from build123d import *

# Parameters (mm, degrees)
F0_R          = 1.55
F1_DEPTH      = 3
F2_SIZE2      = 2.99999
F2_SIZE       = 0.49999
F2_2_SIZE2    = 2.99999
F2_2_SIZE     = 0.49999
F4_DEPTH      = 6
F5_DEPTH      = 6
F6_R          = 1.5
F7_DEPTH      = 25
F9_W          = 5.3
F9_H          = 30.2732266598
F10_DEPTH     = 25
F11_R         = 4
F12_T4_DEPTH  = 20.5670004785
F12_T10_DEPTH = 20.5670004785
F12_T16_DEPTH = 20.5670004785
F12_T22_DEPTH = 20.5670004785
F13_SIZE      = 0.2


# Not quite as in the source:
# - a fillet or chamfer that OpenCascade refuses, or shapes differently, is made with other operations: its cross-section is extruded or revolved along the edge and cut away or added
# - a fillet or chamfer is up to 0.001 mm smaller than in the source, because OpenCascade refuses the exact size
# - ends of sketch curves that miss each other by under 0.0002 mm in the source are joined


with BuildPart() as f1:
    # F0 (on Front) → F1 (new body)
    with BuildSketch(Plane.XZ):
        with BuildLine():
            Line((-17.1, 5.6), (-17.1, -5.6))
            Line((-17.1, -5.6), (17.1, -5.6))
            Line((17.1, -5.6), (17.1, 5.6))
            Line((17.1, 5.6), (9.1844569534, 5.6))
            add(Edge.make_bspline(
                [(9.1844569534, 5.6), (9.1844569534, 2.9670004785), (9.1844569534, 2.9670004785), (-0.0155430466, 2.9670004785)],
                knots=[0, 0, 0, 0, 9.5693619495, 9.5693619495, 9.5693619495, 9.5693619495], degree=3))
            add(Edge.make_bspline(
                [(-9.2155430466, 5.6), (-9.2155430466, 2.9670004785), (-9.2155430466, 2.9670004785), (-0.0155430466, 2.9670004785)],
                knots=[0, 0, 0, 0, 9.5693618638, 9.5693618638, 9.5693618638, 9.5693618638], degree=3))
            Line((-9.2155430466, 5.6), (-17.1, 5.6))
        make_face()
        with Locations((-13, 0)):
            Circle(F0_R, mode=Mode.SUBTRACT)
        with Locations((13, 0)):
            Circle(F0_R, mode=Mode.SUBTRACT)
    extrude(amount=F1_DEPTH)

    # F2 (size 0.5 and 3 in the source; OpenCascade refuses exactly that, so slightly less here)
    f2_edges = [f1.edges().sort_by_distance(p)[0] for p in [
        (-13.157772, 0, 5.6),
        (13.142228, 0, 5.6),
    ]]
    f2_side = f1.faces().sort_by_distance((0.002222, 0, -0.619959))[0]
    chamfer(f2_edges, length=F2_SIZE, length2=F2_SIZE2, reference=f2_side)

    # F2#2 (size 0.5 and 3 in the source; OpenCascade refuses exactly that, so slightly less here)
    f2_2_edges = [f1.edges().sort_by_distance(p)[0] for p in [
        (0, -3, -5.6),
    ]]
    f2_2_side = f1.faces().sort_by_distance((0.002222, -3, -0.619959))[0]
    chamfer(f2_2_edges, length=F2_2_SIZE, length2=F2_2_SIZE2, reference=f2_2_side)

    # F3 (on Right) → F4 (join)
    with BuildSketch(Plane.YZ):
        Polygon((-33.2732266598, 2.4479631427), (-3, -5.1), (-3, 2.9670004785), (-4.2113326633, 3.2690196322), (-4.1453789697, 3.5335454488), (-31.3136593055, 10.3073585255), align=None)
    extrude(amount=F4_DEPTH)

    # F5 (add): a face of the model
    f5_faces = [f1.faces().sort_by_distance(p)[0] for p in [
        (0, -17.6712487641, 2.6798726591),
    ]]
    extrude(f5_faces, amount=F5_DEPTH)

    # F6 (on face) → F7 (cut)
    with BuildSketch(Plane.YZ.offset(6)):
        with Locations((-27.4419643513, 5.1680513561)):
            Circle(F6_R)
        with Locations((-17.7390070885, 2.7488324001)):
            Circle(F6_R)
        with Locations((-12.8875284571, 1.5392229221)):
            Circle(F6_R)
        with Locations((-8.0360498257, 0.3296134441)):
            Circle(F6_R)
    extrude(amount=-F7_DEPTH, mode=Mode.SUBTRACT)

    # F9 (on face) → F10 (cut)
    with BuildSketch(Plane(origin=(0, 0, -5.6), x_dir=(1, 0, 0), z_dir=(0, 0, -1))):
        with Locations((0, 18.1366133299)):
            Rectangle(F9_W, F9_H)
    extrude(amount=-F10_DEPTH, mode=Mode.SUBTRACT)

    # F11
    f11_edges = [f1.edges().sort_by_distance(p)[0] for p in [
        (-4.325, -33.273227, 2.447963),
        (4.325, -33.273227, 2.447963),
        (-4.325, -31.313659, 10.307359),
        (4.325, -31.313659, 10.307359),
    ]]
    fillet(f11_edges, radius=F11_R)

    # F12: fillet of radius 2.5 on 2 edges, made by hand


with BuildPart() as f12_tool2:
    # F12_s3 → F12_t4 (new body)
    with BuildSketch(Plane.XY.offset(-11.35)):
        with BuildLine():
            ThreePointArc((-0.15, -3), (-1.917766953, -3.732233047), (-2.65, -5.5))
            Line((-2.65, -5.5), (-2.65, -3))
            Line((-2.65, -3), (-0.15, -3))
        make_face()
    extrude(amount=F12_T4_DEPTH)

    split(bisect_by=Plane(origin=(0, 0.520882565, 2.0891458603), x_dir=(1, 0, 0), z_dir=(0, -0.2419218956, -0.9702957263)), keep=Keep.TOP)

    split(bisect_by=Plane(origin=(0, -1.3727310958, -5.505723706), x_dir=(1, 0, 0), z_dir=(0, 0.2419218956, 0.9702957263)), keep=Keep.TOP)


with BuildPart() as f1_1:
    add(f1.part)

    # F12_t1: union F12_tool2
    add(f12_tool2.part)


with BuildPart() as f12_tool8:
    # F12_s9 → F12_t10 (new body)
    with BuildSketch(Plane.XY.offset(-11.35)):
        with BuildLine():
            ThreePointArc((-0.15, -3), (-1.917766953, -3.732233047), (-2.65, -5.5))
            Line((-2.65, -5.5), (-2.65, -3))
            Line((-2.65, -3), (-0.15, -3))
        make_face()
    extrude(amount=F12_T10_DEPTH)

    split(bisect_by=Plane(origin=(0, -4.7322152283, 1.1798737719), x_dir=(1, 0, 0), z_dir=(0, -0.9702957263, 0.2419218956)), keep=Keep.TOP)

    split(bisect_by=Plane(origin=(0, 0.5868362585, 2.3536716769), x_dir=(1, 0, 0), z_dir=(0, -0.2419218956, -0.9702957263)), keep=Keep.TOP)


with BuildPart() as f1_2:
    add(f1_1.part)

    # F12_t7: union F12_tool8
    add(f12_tool8.part)


with BuildPart() as f12_tool14:
    # F12_s15 → F12_t16 (new body)
    with BuildSketch(Plane.XY.offset(-11.35)):
        with BuildLine():
            ThreePointArc((0.15, -3), (1.917766953, -3.732233047), (2.65, -5.5))
            Line((2.65, -5.5), (2.65, -3))
            Line((2.65, -3), (0.15, -3))
        make_face()
    extrude(amount=F12_T16_DEPTH)

    split(bisect_by=Plane(origin=(0, -1.3727310958, -5.505723706), x_dir=(1, 0, 0), z_dir=(0, 0.2419218956, 0.9702957263)), keep=Keep.TOP)

    split(bisect_by=Plane(origin=(0, 0.520882565, 2.0891458603), x_dir=(1, 0, 0), z_dir=(0, -0.2419218956, -0.9702957263)), keep=Keep.TOP)


with BuildPart() as f1_3:
    add(f1_2.part)

    # F12_t13: union F12_tool14
    add(f12_tool14.part)


with BuildPart() as f12_tool20:
    # F12_s21 → F12_t22 (new body)
    with BuildSketch(Plane.XY.offset(-11.35)):
        with BuildLine():
            ThreePointArc((0.15, -3), (1.917766953, -3.732233047), (2.65, -5.5))
            Line((2.65, -5.5), (2.65, -3))
            Line((2.65, -3), (0.15, -3))
        make_face()
    extrude(amount=F12_T22_DEPTH)

    split(bisect_by=Plane(origin=(0, -4.7322152283, 1.1798737719), x_dir=(1, 0, 0), z_dir=(0, -0.9702957263, 0.2419218956)), keep=Keep.TOP)

    split(bisect_by=Plane(origin=(0, 0.5868362585, 2.3536716769), x_dir=(1, 0, 0), z_dir=(0, -0.2419218956, -0.9702957263)), keep=Keep.TOP)


with BuildPart() as f1_4:
    add(f1_3.part)

    # F12_t19: union F12_tool20
    add(f12_tool20.part)

    # F13
    f13_edges = [f1_4.edges().sort_by_distance(p)[0] for p in [
        (4.125595, -4.145379, 3.533545),
        (-4.125595, -4.145379, 3.533545),
    ]]
    chamfer(f13_edges, length=F13_SIZE)


solid = f1_4.part
Check sheet for the modelled part. Datum: model origin and axes. Units: mm. A direction names the side the tool comes from. Round coordinates to 2 decimals unless told otherwise and drop trailing zeros. Order: outer loops, then holes, each group sorted by start corner. A loop starts at its lowest first (then second) coordinate and runs counter-clockwise, first axis right, second up.
(1) Scan lines: probe 1 along Y at (x, z) = (-3.5, 2) (3 decimals); probe 2 along X at (y, z) = (-22, 0.25); probe 3 along Y at (x, z) = (12, 2.25). Record each from-to range of solid material in increasing order.
(2) Cross-section at C-C, the plane z = 8.75. Enter the section's corners in (x, y).
(3) Draft check along X on faces 1 (the flat face through (-0.239, -1.479, -5.354)), 2 (the cylindrical face through (11.45, -1.48, 0.07)). Enter one of: pulls with the +X half, pulls with the -X half, needs draft (parallel to the pull), parting line crosses it, or undercut.
(4) Go/stop test with flat-tipped pins: P1, Ø5, axis at y = -8.04, z = 0.33, coming from the -X side; P2, Ø2.5, axis at y = -8.04, z = 0.33, coming from the +X side; P3, Ø4.5, axis at y = -15.5, z = 0, coming from the +X side; P4, Ø8.5, axis at x = -2, z = 1, coming from the -Y side. Record where each tip stops, or that it passes through.
(5) Cross-section at B-B, the plane y = -23.5. Enter the section's corners in (x, z).
(6) Access from +Z, -Z, +X, -X, +Y, -Y to the whole of each face (thin tool, end or side, straight path). Record for faces 3 (the flat face through (-2.65, -19, 4)), 4 (the cylindrical face through (4.35, -26.01, 5.62)).
Check sheet entries:
1. probe 1: y = -30.592 to -19.039, -16.439 to -14.315, -11.46 to 0
1. probe 2: x = -6 to -2.65, 2.65 to 6
1. probe 3: y = -3 to 0
2. outline: (-6, -30.67) - (-2.65, -30.67) - (-2.65, -25.07) - (-6, -25.07) - close; (2.65, -30.67) - (6, -30.67) - (6, -25.07) - (2.65, -25.07) - close
3. face 1: needs draft
3. face 2: undercut
4. P1: stops at x = -6
4. P2: passes through
4. P3: stops at x = 6
4. P4: stops at y = -32.42
5. outline: (-6, 0.01) - (-2.65, 0.01) - (-2.65, 8.36) - (-6, 8.36) - close; (2.65, 0.01) - (6, 0.01) - (6, 8.36) - (2.65, 8.36) - close
6. face 3: +Z, -Z, -Y
6. face 4: +X, -X
